Work out the finished part from the listing and answer in its coordinate system (mm). A direction names the side the tool comes from. Round coordinates to 2 decimals unless told otherwise and drop trailing zeros. Write each loop counter-clockwise with the first axis right and the second up, starting at its lowest first coordinate (ties: lowest second). Pieces come first, ordered by that corner, then holes. Notation, with made-up numbers: (89.25, -21) -> (145.25, -21) arc R30 ccw to (145.25, 3) -> close; hole circle Ø5 at (43, 53.25). An arc over 180 degrees is marked (long way). Answer as a JSON object with one key per item and string values. Group by question number.
from build123d import *

# Parameters (mm, degrees)
EXTRUDE_1_DEPTH      = 57
SKETCH_2_W           = 35
SKETCH_2_H           = 10
CUT_EXTRUDE_1_DEPTH  = 90.319650693
CUT_EXTRUDE_2_REACH  = 94.32
SKETCH_3_R           = 20.1
SKETCH_4_R           = 4.5
CUT_EXTRUDE_6_DEPTH  = 2
CUT_EXTRUDE_7_REACH  = 94.32
SKETCH_5_R           = 2.5
CUT_EXTRUDE_8_REACH  = 94.32
SKETCH_9_R           = 10.1
CUT_EXTRUDE_9_REACH  = 94.32
SKETCH_1786_R        = 1.6
SKETCH_12_R          = 3.1
CUT_EXTRUDE_10_DEPTH = 3


with BuildPart() as part:
    # 草图1 → 凸台-拉伸1 (new body)
    with BuildSketch(Plane.XY):
        Polygon((0, 0), (0, 57), (5, 57), (5, 5), (40, 5), (40, 57), (45, 57), (45, 0), align=None)
    extrude(amount=EXTRUDE_1_DEPTH)

    # 草图2 → 切除-拉伸1 (cut, through all)
    with BuildSketch(Plane(origin=(0, 5, 0), x_dir=(1, 0, 0), z_dir=(0, 1, 0))):
        with Locations((22.5, -52)):
            Rectangle(SKETCH_2_W, SKETCH_2_H)
        with Locations((22.5, -5)):
            Rectangle(SKETCH_2_W, SKETCH_2_H)
    extrude(amount=-CUT_EXTRUDE_1_DEPTH, mode=Mode.SUBTRACT)

    # 草图3 → 切除-拉伸2 (cut, up to next)
    with BuildSketch(Plane.ZY, mode=Mode.PRIVATE) as cut_extrude_2_sk1:
        with Locations((28.5, 28.5)):
            Circle(SKETCH_3_R)
    cut_extrude_2_tool1 = extrude(cut_extrude_2_sk1.sketch, amount=-CUT_EXTRUDE_2_REACH, mode=Mode.PRIVATE) & part.part
    add(cut_extrude_2_tool1.solids().sort_by_distance((0, 28.5, 28.5))[0], mode=Mode.SUBTRACT)

    # 草图4 → 切除-拉伸6 (cut)
    with BuildSketch(Plane(origin=(5, 0, 0), x_dir=(0, 0, -1), z_dir=(1, 0, 0))):
        with Locations(Location((-52, 52, 0), (0, 0, 90))):
            Circle(SKETCH_4_R)
        with Locations(Location((-5, 52, 0), (0, 0, 90))):
            Circle(SKETCH_4_R)
        with Locations(Location((-5, 5, 0), (0, 0, 90))):
            Circle(SKETCH_4_R)
        with Locations(Location((-52, 5, 0), (0, 0, 90))):
            Circle(SKETCH_4_R)
    extrude(amount=-CUT_EXTRUDE_6_DEPTH, mode=Mode.SUBTRACT)

    # 草图5 → 切除-拉伸7 (cut, up to next)
    with BuildSketch(Plane(origin=(0, 0, 0), x_dir=(0, 0, -1), z_dir=(1, 0, 0)), mode=Mode.PRIVATE) as cut_extrude_7_sk1:
        with Locations(Location((-52, 52, 0), (0, 0, 90))):
            Circle(SKETCH_5_R)
    cut_extrude_7_tool1 = extrude(cut_extrude_7_sk1.sketch, amount=CUT_EXTRUDE_7_REACH, mode=Mode.PRIVATE) & part.part
    # 草图5 → 切除-拉伸7 (cut, up to next)
    with BuildSketch(Plane(origin=(0, 0, 0), x_dir=(0, 0, -1), z_dir=(1, 0, 0)), mode=Mode.PRIVATE) as cut_extrude_7_sk2:
        with Locations(Location((-5, 52, 0), (0, 0, 90))):
            Circle(SKETCH_5_R)
    cut_extrude_7_tool2 = extrude(cut_extrude_7_sk2.sketch, amount=CUT_EXTRUDE_7_REACH, mode=Mode.PRIVATE) & part.part
    # 草图5 → 切除-拉伸7 (cut, up to next)
    with BuildSketch(Plane(origin=(0, 0, 0), x_dir=(0, 0, -1), z_dir=(1, 0, 0)), mode=Mode.PRIVATE) as cut_extrude_7_sk3:
        with Locations(Location((-5, 5, 0), (0, 0, 90))):
            Circle(SKETCH_5_R)
    cut_extrude_7_tool3 = extrude(cut_extrude_7_sk3.sketch, amount=CUT_EXTRUDE_7_REACH, mode=Mode.PRIVATE) & part.part
    # 草图5 → 切除-拉伸7 (cut, up to next)
    with BuildSketch(Plane(origin=(0, 0, 0), x_dir=(0, 0, -1), z_dir=(1, 0, 0)), mode=Mode.PRIVATE) as cut_extrude_7_sk4:
        with Locations(Location((-52, 5, 0), (0, 0, 90))):
            Circle(SKETCH_5_R)
    cut_extrude_7_tool4 = extrude(cut_extrude_7_sk4.sketch, amount=CUT_EXTRUDE_7_REACH, mode=Mode.PRIVATE) & part.part
    add(cut_extrude_7_tool1.solids().sort_by_distance((0, 52, 52))[0], mode=Mode.SUBTRACT)
    add(cut_extrude_7_tool2.solids().sort_by_distance((0, 52, 5))[0], mode=Mode.SUBTRACT)
    add(cut_extrude_7_tool3.solids().sort_by_distance((0, 5, 5))[0], mode=Mode.SUBTRACT)
    add(cut_extrude_7_tool4.solids().sort_by_distance((0, 5, 52))[0], mode=Mode.SUBTRACT)

    # 草图9 → 切除-拉伸8 (cut, up to next)
    with BuildSketch(Plane(origin=(45, 0, 0), x_dir=(0, 0, -1), z_dir=(1, 0, 0)), mode=Mode.PRIVATE) as cut_extrude_8_sk1:
        with Locations(Location((-28.5, 28.5, 0), (0, 0, 90))):
            Circle(SKETCH_9_R)
    cut_extrude_8_tool1 = extrude(cut_extrude_8_sk1.sketch, amount=-CUT_EXTRUDE_8_REACH, mode=Mode.PRIVATE) & part.part
    add(cut_extrude_8_tool1.solids().sort_by_distance((45, 28.5, 28.5))[0], mode=Mode.SUBTRACT)

    # Sketch 1786 → 切除-拉伸9 (cut, up to next)
    with BuildSketch(Plane(origin=(45, 0, 0), x_dir=(0, 0, -1), z_dir=(1, 0, 0)), mode=Mode.PRIVATE) as cut_extrude_9_sk1:
        with Locations(Location((-28.5, 13.5, 0), (0, 0, 90))):
            Circle(SKETCH_1786_R)
    cut_extrude_9_tool1 = extrude(cut_extrude_9_sk1.sketch, amount=-CUT_EXTRUDE_9_REACH, mode=Mode.PRIVATE) & part.part
    # Sketch 1786 → 切除-拉伸9 (cut, up to next)
    with BuildSketch(Plane(origin=(45, 0, 0), x_dir=(0, 0, -1), z_dir=(1, 0, 0)), mode=Mode.PRIVATE) as cut_extrude_9_sk2:
        with Locations(Location((-41.490381057, 36, 0), (0, 0, 90))):
            Circle(SKETCH_1786_R)
    cut_extrude_9_tool2 = extrude(cut_extrude_9_sk2.sketch, amount=-CUT_EXTRUDE_9_REACH, mode=Mode.PRIVATE) & part.part
    # Sketch 1786 → 切除-拉伸9 (cut, up to next)
    with BuildSketch(Plane(origin=(45, 0, 0), x_dir=(0, 0, -1), z_dir=(1, 0, 0)), mode=Mode.PRIVATE) as cut_extrude_9_sk3:
        with Locations(Location((-15.509618943, 36, 0), (0, 0, 90))):
            Circle(SKETCH_1786_R)
    cut_extrude_9_tool3 = extrude(cut_extrude_9_sk3.sketch, amount=-CUT_EXTRUDE_9_REACH, mode=Mode.PRIVATE) & part.part
    add(cut_extrude_9_tool1.solids().sort_by_distance((45, 13.5, 28.5))[0], mode=Mode.SUBTRACT)
    add(cut_extrude_9_tool2.solids().sort_by_distance((45, 36, 41.490381))[0], mode=Mode.SUBTRACT)
    add(cut_extrude_9_tool3.solids().sort_by_distance((45, 36, 15.509619))[0], mode=Mode.SUBTRACT)

    # 草图12 → 切除-拉伸10 (cut)
    with BuildSketch(Plane.ZY.offset(-40)):
        with Locations((28.5, 13.5)):
            Circle(SKETCH_12_R)
        with Locations((15.509618943, 36)):
            Circle(SKETCH_12_R)
        with Locations((41.490381057, 36)):
            Circle(SKETCH_12_R)
    extrude(amount=-CUT_EXTRUDE_10_DEPTH, mode=Mode.SUBTRACT)


solid = part.part
1) A cutting plane is placed at C-C on y = 36. State how many separate pieces and enclosed holes the cut face has, plus the area to 3 significant figures.
2) A cutting plane is placed at D-D on z = 52. Determine the outline of the cut face in (x, y), plus the area to 3 significant figures.
3) Each of these flat-tipped pins is pushed along its axis until it touches: P1, Ø10, axis at y = 36, z = 15.51, coming from the -X side; P2, Ø2, axis at x = 28, z = 47, coming from the +Y side; P3, Ø12, axis at y = 6.5, z = 14, coming from the -X side; P4, Ø2.5, axis at x = 14.5, y = 2.5, coming from the -Z side. Where does it stop, or does it pass through?
4) A cutting plane is placed at B-B on z = 28.5. Determine the outline of the cut face in (x, y).
5) A tool of negligible diameter and unlimited length cuts with its end or side. For faces 1 (the face through (22, 5, 28)), 2 (the face through (22, 3, 47)), 3 (the face through (41.5, 13.6, 25.4)), 4 (the face through (4.01, 7.08, 1.01)), from which of +Z, -Z, +X, -X, +Y, -Y can it reach the whole face along a straight path? Write none if from no direction.
6) A cutting plane is placed at A-A on y = 28.5. Determine the outline of the cut face in (x, z), plus the area to 3 significant figures.
7) Straight lines are drawn through the part: L1, parallel to Y at x = 1.7, z = 5; L2, parallel to X at y = 53.5, z = 26. For each, find the intervals that lie inside material, in ascending order.
8) For a pull along Z with two mould halves and no side action, classify faces 5 (the face through (3, 29, 57)), 6 (the face through (2, 57, 28)), 7 (the face through (41.479, 39.074, 15.106)) as released by +Z, released by -Z, zero draft, split by the parting line, or undercut.
Established:
{
 "1": {"separate pieces": "6", "enclosed holes": "0", "area": "266 mm²"},
 "2": {"outline": "(0, 0) -> (5, 0) -> (5, 0.5) -> (3, 0.5) -> (3, 2.5) -> (0, 2.5) -> close; (0, 7.5) -> (3, 7.5) -> (3, 9.5) -> (5, 9.5) -> (5, 47.5) -> (3, 47.5) -> (3, 49.5) -> (0, 49.5) -> close; (0, 54.5) -> (3, 54.5) -> (3, 56.5) -> (5, 56.5) -> (5, 57) -> (0, 57) -> close; (40, 0) -> (45, 0) -> (45, 57) -> (40, 57) -> close", "area": "504 mm²"},
 "3": {"P1": "stops at x = 40", "P2": "stops at y = 5", "P3": "stops at x = 0", "P4": "stops at z = 10"},
 "4": {"outline": "(0, 0) -> (45, 0) -> (45, 11.9) -> (43, 11.9) -> (43, 10.4) -> (40, 10.4) -> (40, 5) -> (5, 5) -> (5, 8.4) -> (0, 8.4) -> close; (0, 48.6) -> (5, 48.6) -> (5, 57) -> (0, 57) -> close; (40, 16.6) -> (43, 16.6) -> (43, 15.1) -> (45, 15.1) -> (45, 18.4) -> (40, 18.4) -> close; (40, 38.6) -> (45, 38.6) -> (45, 57) -> (40, 57) -> close"},
 "5": {"face 1": "+Z, -Z, +Y", "face 2": "+Z, +Y, -Y", "face 3": "-X", "face 4": "none"},
 "6": {"outline": "(0, 0) -> (5, 0) -> (5, 8.4) -> (0, 8.4) -> close; (0, 48.6) -> (5, 48.6) -> (5, 57) -> (0, 57) -> close; (40, 0) -> (45, 0) -> (45, 18.4) -> (40, 18.4) -> close; (40, 38.6) -> (45, 38.6) -> (45, 57) -> (40, 57) -> close", "area": "268 mm²"},
 "7": {"L1": "y = 0 to 2.5, 7.5 to 49.5, 54.5 to 57", "L2": "x = 0 to 5, 40 to 45"},
 "8": {"face 5": "released by +Z", "face 6": "zero draft", "face 7": "undercut"}
}
